Here's the drawing with two shaded views (mm, measured from the low corner). I have some questions. Coordinates: 2 decimals unless noted, no trailing zeros. Write each loop counter-clockwise with the first axis right and the second up, starting at its lowest first coordinate (ties: lowest second). Pieces come first, ordered by that corner, then holes. Notation, with made-up numbers: (-15.5, 24) -> (31.5, 24) arc R14 ccw to (31.5, 33) -> close; hole circle Ø9 at (-29.75, 73.5). An arc over 180 degrees is marked (long way). Put each result on its own line as item: value. Start each with the question number.
Item 1: I need wall thicknesses on line 1 (Z direction, x = 101.6, y = 4.25). Which ranges of the line are inside material? Lowest first, please. Write a range as [from, to].
Item 2: I want a section at A-A, the plane z = 6.35. State how many separate pieces and enclosed holes the cut face has, then the cut area to 3 significant figures.
Item 3: If we mould it in two halves opening along Y, with no side actions, what happens to the marked faces 1, 2 and 3? For each: released by +Y, released by -Y, zero draft, split by the parting line, or undercut.
Item 4: For pin 1 (5.5 mm diameter, centred on x = 91.28, z = 6.35, fed in from -Y), with a flat end and sliding along its axis, tell me the tip position at first contact or that it passes through.
Item 5: I want a section at C-C, the plane x = 12.7. List the corners of the cut face in (y, z) for me.
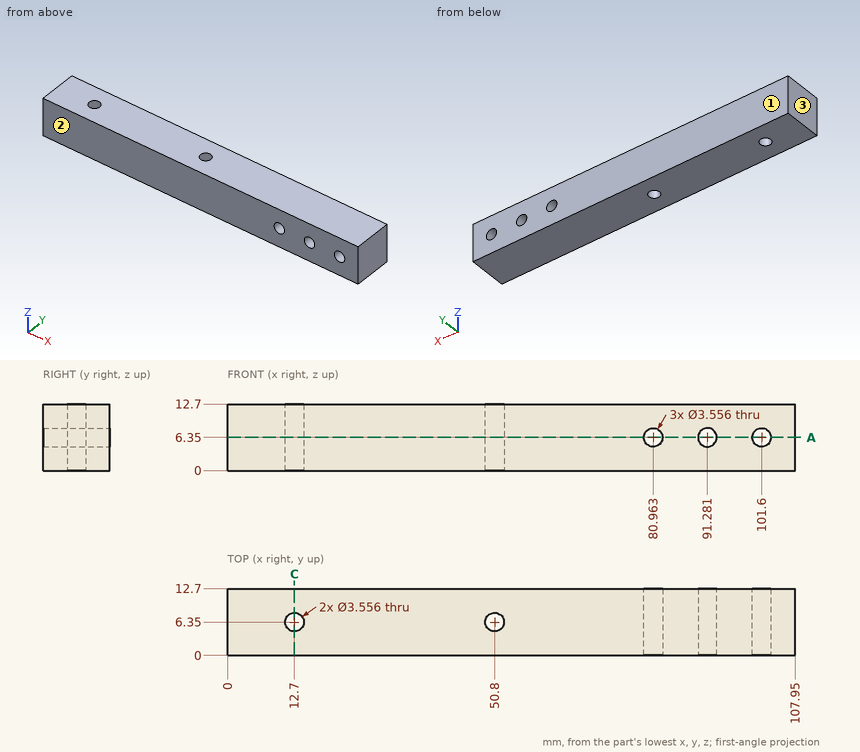
Calculated:
1. line 1: z = [0, 4.57], [8.13, 12.7]
2. separate pieces: 4
2. enclosed holes: 2
2. area: 1,220 mm2
3. face 1: released by +Y
3. face 2: released by -Y
3. face 3: zero draft
4. pin 1: stops at y = 0
5. outline: (0, 0) -> (4.57, 0) -> (4.57, 12.7) -> (0, 12.7) -> close; (8.13, 0) -> (12.7, 0) -> (12.7, 12.7) -> (8.13, 12.7) -> close
